Part print with two shaded views. Sizes in mm from the minimum x, y, z corner. A direction names the side the tool comes from. Give positions to 0.01 mm unless a question says otherwise; leave off trailing zeros. Order: outer loops, then holes, each group sorted by start corner. A loop starts at its lowest first (then second) coordinate and runs counter-clockwise, first axis right, second up. Notation, with made-up numbers: M 74,0 L 119,0 A14 ccw 119,20 Z; hole C 7,-19 d7. An arc over 180 degrees is marked long. Return JSON: item names as keys, results as strings.
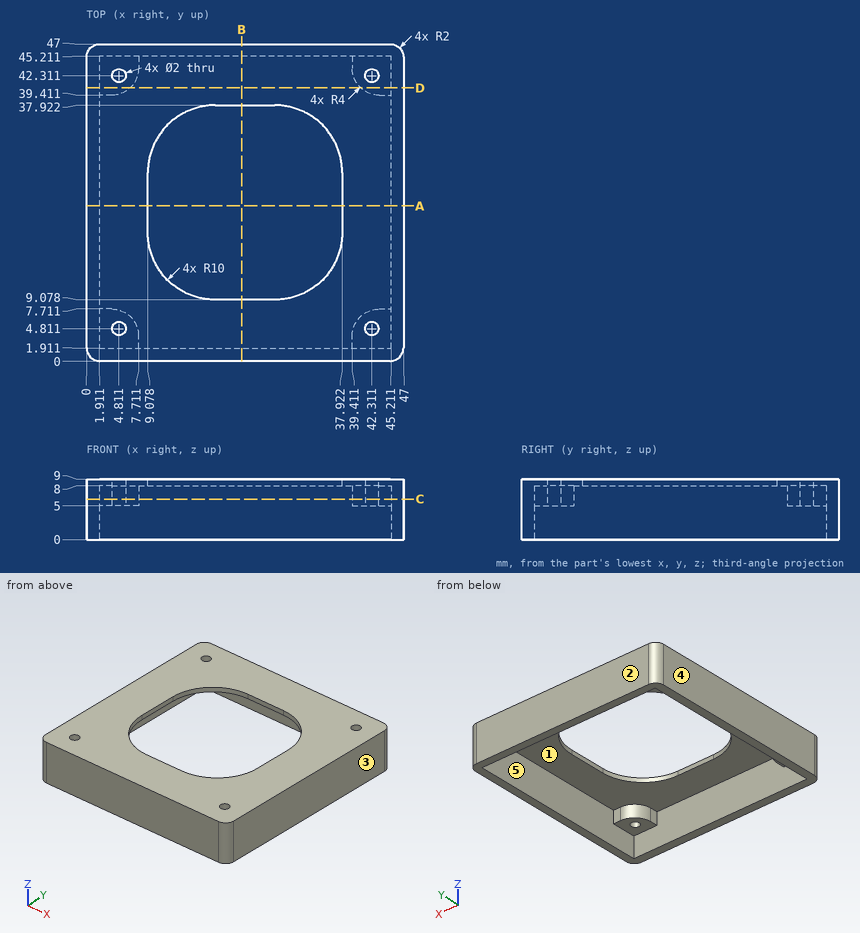
Q1. Band-saw the part on C-C (z = 6). Give the cut face in (x, y).
Established:
{"outline": "M 0,2 A2 ccw 2,0 L 45,0 A2 ccw 47,2 L 47,45 A2 ccw 45,47 L 2,47 A2 ccw 0,45 Z; hole M 1.91,7.71 L 3.71,7.71 A4 cw 7.71,3.71 L 7.71,1.91 L 39.41,1.91 L 39.41,3.71 A4 cw 43.41,7.71 L 45.21,7.71 L 45.21,39.41 L 43.41,39.41 A4 cw 39.41,43.41 L 39.41,45.21 L 7.71,45.21 L 7.71,43.41 A4 cw 3.71,39.41 L 1.91,39.41 Z; hole C 4.81,4.81 d2; hole C 4.81,42.31 d2; hole C 42.31,4.81 d2; hole C 42.31,42.31 d2"}
Q2. 3-axis set-ups, long thin cutter, end or side, ignore diameter. For the marked faces 4 and 5: which of +Z, -Z, +X, -X, +Y, -Y reach the whole face in a straight line?
Established:
{"face 4": "+Z, -Z, -X, +Y, -Y", "face 5": "-Z"}
Q3. Two-plate mould, pull along Y, no slides. Class the marked faces 1, 2 and 3: +Y half, -Y half, draft (parallel to the pull), parting line (faces both ways), or undercut.
Established:
{"face 1": "undercut", "face 2": "+Y half", "face 3": "draft"}
Q4. Band-saw the part on D-D (y = 40.5). Give the cut face in (x, z), then the cut area to 3 significant figures.
Established:
{"outline": "M 0,0 L 1.91,0 L 1.91,5 L 6.45,5 L 6.45,8 L 40.67,8 L 40.67,5 L 45.21,5 L 45.21,0 L 47,0 L 47,9 L 0,9 Z", "area": "104 mm²"}
Q5. Band-saw the part on A-A (y = 23). Give the cut face in (x, z).
Established:
{"outline": "M 0,0 L 1.91,0 L 1.91,8 L 9.08,8 L 9.08,9 L 0,9 Z; M 37.92,8 L 45.21,8 L 45.21,0 L 47,0 L 47,9 L 37.92,9 Z"}
Q6. Pin check, flat tips, straight feed: pin 1 (4.5 mm diameter, centred on x = 5.5, y = 6, fed in from -Z); pin 2 (1.5 mm diameter, centred on x = 40, y = 32, fed in from -Z). Stop position of each tip, or through.
Established:
{"pin 1": "stops at z = 5", "pin 2": "stops at z = 8"}
Q7. Probe line 1 along Y through (x, z) = (19, 7); line 2 along X through (y, z) = (4.5, 5.75). List the from-to ranges inside material, lowest first.
Established:
{"line 1": "y = 0 to 1.91, 45.21 to 47", "line 2": "x = 0 to 3.86, 5.76 to 7.63, 39.49 to 41.36, 43.26 to 47"}
